Answer from the drawing. Dimensions are ordinates in mm from the lowest x, y and z of the part. A direction names the side the tool comes from. Round coordinates to 2 decimals unless told otherwise and drop trailing zeros. Order: outer loops, then holes, each group sorted by start corner. A loop starts at its lowest first (then second) coordinate and runs counter-clockwise, first axis right, second up. Notation, with made-up numbers: (-29.75, 89) -> (-12.75, 89) arc R15 ccw to (-12.75, 106) -> close; hole circle Ø4 at (87, 12). An arc over 180 degrees is marked (long way). Use a Markdown table: item, result. Add a question column.
1. Section B-B, the plane x = 5 is taken. Give the vertices of the cut face in (y, z).
2. Section D-D, the plane z = 2 is taken. Give the vertices of the cut face in (x, y).
3. Section A-A, the plane z = 5 is taken. Give the vertices of the cut face in (x, y), then the cut area to 3 significant figures.
4. For the marked faces 1 and 2, determine the directions among +Z, -Z, +X, -X, +Y, -Y from which every point of the face is accessible in a straight line to the end or side of a thin tool.
5. Section C-C, the plane y = 4.5 is taken. Give the vertices of the cut face in (x, z).
6. Given pin 1 (2 mm diameter, centred on x = 5, z = 2.5, fed in from -Y); pin 2 (2.5 mm diameter, centred on x = 5, z = 5, fed in from -Y); pin 3 (3 mm diameter, centred on y = 2.5, z = 3.5, fed in from -X); pin 4 (1 mm diameter, centred on x = 2, y = 2.5, fed in from +Z), each flat-ended and moving along its own axis, determine where each tip first touches the part or whether it passes through.
7. Consider L1, parallel to X at y = 1.9, z = 5; L2, parallel to X at y = 1.45, z = 5. Determine where each line is inside the solid, lowest interval first. Write a range as [from, to].
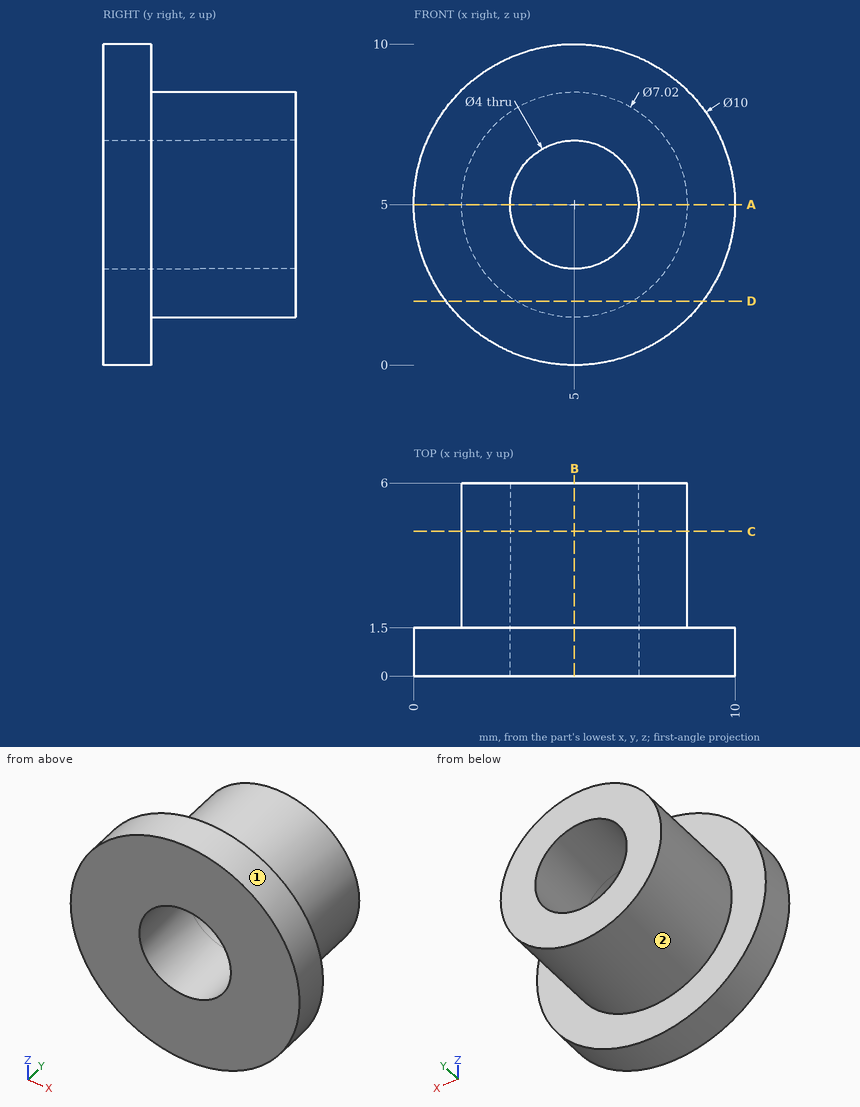
Verdict:
| question | item | result |
|---|---|---|
| 1 | outline | (0, 0) -> (1.5, 0) -> (1.5, 1.49) -> (6, 1.49) -> (6, 3) -> (0, 3) -> close; (0, 7) -> (6, 7) -> (6, 8.51) -> (1.5, 8.51) -> (1.5, 10) -> (0, 10) -> close |
| 2 | outline | (1, 0) -> (9, 0) -> (9, 1.5) -> (6.82, 1.5) -> (6.82, 6) -> (3.18, 6) -> (3.18, 1.5) -> (1, 1.5) -> close |
| 3 | outline | (0, 0) -> (3, 0) -> (3, 6) -> (1.49, 6) -> (1.49, 1.5) -> (0, 1.5) -> close; (7, 0) -> (10, 0) -> (10, 1.5) -> (8.51, 1.5) -> (8.51, 6) -> (7, 6) -> close |
| 3 | area | 22.6 mm2 |
| 4 | face 1 | +Y, -Y |
| 4 | face 2 | +Y |
| 5 | outline | circle Ø7.02 at (5, 5); hole circle Ø4 at (5, 5) |
| 6 | pin 1 | stops at y = 0 |
| 6 | pin 2 | passes through |
| 6 | pin 3 | stops at x = 0.01 |
| 6 | pin 4 | stops at z = 7.46 |
| 7 | L1 | x = [1.49, 3], [7, 8.51] |
| 7 | L2 | x = [0, 3], [7, 10] |
